Print and shaded views of the part. All mm, measured from the part's lowest x, y and z. A direction names the side the tool comes from. Give positions to 0.01 mm unless a question says otherwise; leave off trailing zeros. Order: outer loops, then holes, each group sorted by start corner. A loop starts at its lowest first (then second) coordinate and runs counter-clockwise, first axis right, second up. Notation, with made-up numbers: (65.5, -13.5) - (72.5, -13.5) arc R19 cw to (72.5, 13.5) - close; hole circle Ø7 at (29, -35.5). An arc over 180 degrees is marked (long way). Answer in a Markdown table with one row per item.
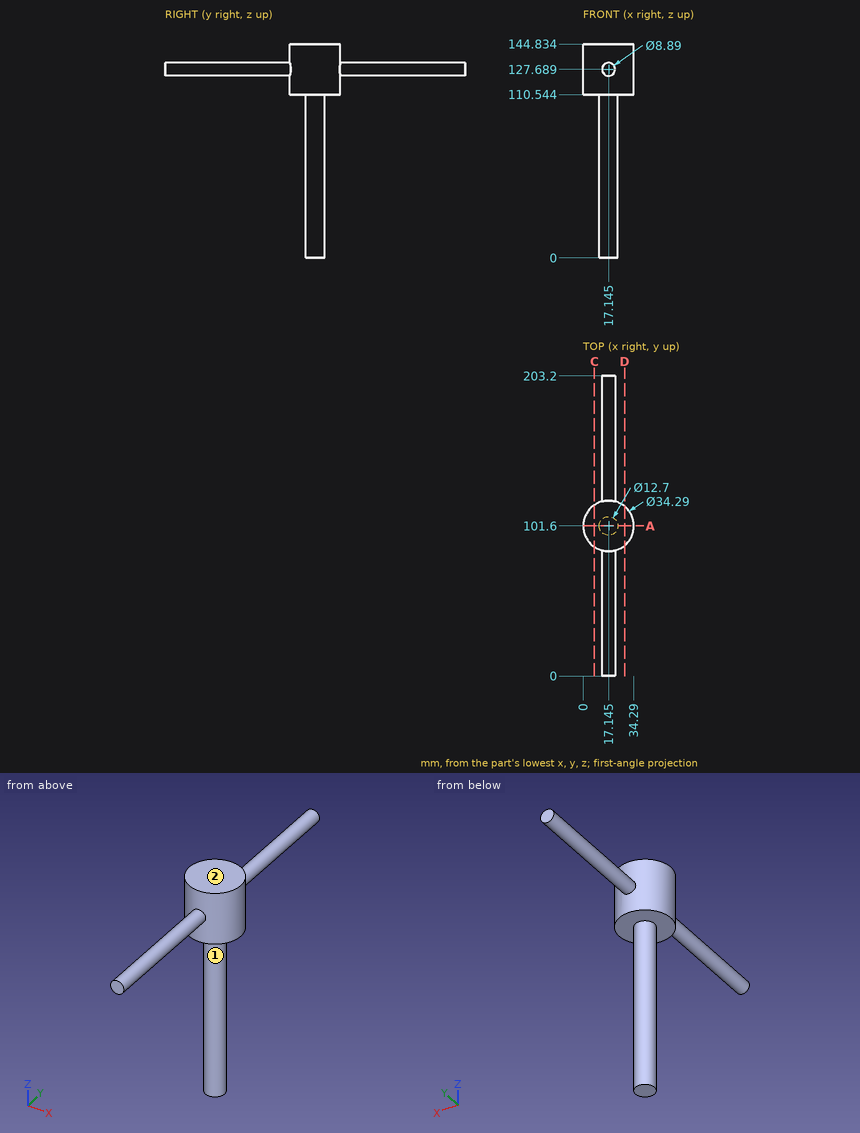
1. Probe line 1 (Z direction, x = 11, y = 117.5) (1 decimal); line 2 (Y direction, x = 8, z = 126); line 3 (Z direction, x = 19.5, y = 164). List the from-to ranges inside material, lowest first.
Check result:
| item | result |
|---|---|
| line 1 | z = 110.5 to 144.8 |
| line 2 | y = 87.1 to 116.1 |
| line 3 | z = 123.92 to 131.46 |
2. Drop flat-ended pins along their axis: P1, Ø4, axis at x = 16.5, y = 139, coming from the +Z side; P2, Ø12, axis at x = 4.5, y = 145.5, coming from the -Z side; P3, Ø5, axis at x = 18, z = 43, coming from the +Y side; P4, Ø1.5, axis at x = 15.5, y = 156.5, coming from the +Z side. Give the stop position or say it passes through.
Check result:
| item | result |
|---|---|
| P1 | stops at z = 132.13 |
| P2 | passes through |
| P3 | stops at y = 107.95 |
| P4 | stops at z = 132.04 |
3. Cut at D-D on x = 28. Write the cut outline in (y, z) (1 decimal).
Check result:
| item | result |
|---|---|
| outline | (88.3, 110.5) - (114.9, 110.5) - (114.9, 144.8) - (88.3, 144.8) - close |
4. Cut at A-A on y = 101.6. Write the cut outline in (x, z) (1 decimal), and give its area (3 significant figures).
Check result:
| item | result |
|---|---|
| outline | (0, 110.5) - (10.8, 110.5) - (10.8, 0) - (23.5, 0) - (23.5, 110.5) - (34.3, 110.5) - (34.3, 144.8) - (0, 144.8) - close |
| area | 2,580 mm² |
5. Cut at C-C on x = 7.5. Write the cut outline in (y, z) (1 decimal), and give its area (3 significant figures).
Check result:
| item | result |
|---|---|
| outline | (87.4, 110.5) - (115.8, 110.5) - (115.8, 144.8) - (87.4, 144.8) - close |
| area | 972 mm² |
6. Which spindle directions (+Z, -Z, +X, -X, +Y, -Y) get a long thin tool onto all of the face, cutting with end or side? Do the marked faces 1 and 2. Say none if no direction does.
Check result:
| item | result |
|---|---|
| face 1 | -Z |
| face 2 | +Z, +X, -X, +Y, -Y |
